Source: three-view drawing plus pictorial views. Frame: mm from the lowest corner of the part. Give positions to 0.01 mm unless a question says otherwise; leave off trailing zeros. Order: outer loops, then holes, each group sorted by start corner. A loop starts at its lowest first (then second) coordinate and runs counter-clockwise, first axis right, second up. Notation, with made-up numbers: (63, 10) - (109, 10) arc R28 cw to (109, 30) - close; hole circle Ø5 at (48, 86.25). An arc over 180 degrees is marked (long way). Answer in a Markdown table with one row per item. Add a question column.
1. Section query C-C on x = 45. Return loops of the section in (y, z).
2. Ray query, line 1 (X direction, y = 7.25, z = 45); line 2 (X direction, y = 2.75, z = 6.5). Return the intervals inside material, ascending. Write a range as [from, to].
3. Section query A-A on z = 27. Return loops of the section in (x, y), and give its area (3 significant figures).
4. Mould query, pull axis X, two halves, no side actions, for the marked faces 1, 2 and 3. Classes: released by +X, released by -X, zero draft, split by the parting line, or undercut.
5. Section query B-B on y = 3. Count the separate pieces of the cut face and the enclosed holes in it, and give its area (3 significant figures).
6. Contact query for a flat-ended pin moving along its axis: pin 1 (5.5 mm diameter, centred on x = 45, z = 45, fed in from +Y). Output: stop coordinate, or through.
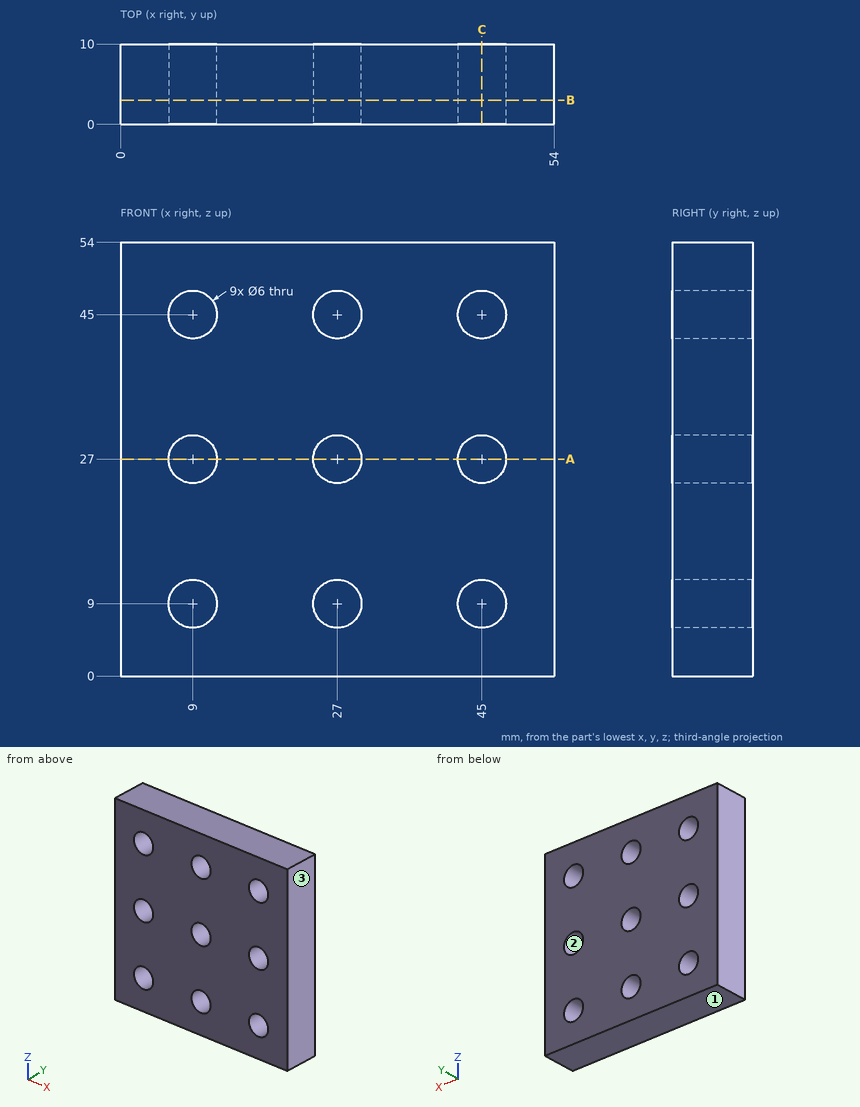
Answer:
| question | item | result |
|---|---|---|
| 1 | outline | (0, 0) - (10, 0) - (10, 6) - (0, 6) - close; (0, 12) - (10, 12) - (10, 24) - (0, 24) - close; (0, 30) - (10, 30) - (10, 42) - (0, 42) - close; (0, 48) - (10, 48) - (10, 54) - (0, 54) - close |
| 2 | line 1 | x = [0, 6], [12, 24], [30, 42], [48, 54] |
| 2 | line 2 | x = [0, 7.34], [10.66, 25.34], [28.66, 43.34], [46.66, 54] |
| 3 | outline | (0, 0) - (6, 0) - (6, 10) - (0, 10) - close; (12, 0) - (24, 0) - (24, 10) - (12, 10) - close; (30, 0) - (42, 0) - (42, 10) - (30, 10) - close; (48, 0) - (54, 0) - (54, 10) - (48, 10) - close |
| 3 | area | 360 mm² |
| 4 | face 1 | zero draft |
| 4 | face 2 | undercut |
| 4 | face 3 | released by +X |
| 5 | separate pieces | 1 |
| 5 | enclosed holes | 9 |
| 5 | area | 2,660 mm² |
| 6 | pin 1 | passes through |
